```python
from build123d import *

# Parameters (mm, degrees)
F0_W     = 25.4
F0_H     = 127
F1_DEPTH = 12.7
F4_DEPTH = 12.7
F2_R     = 9.525
F5_DEPTH = 152.401


with BuildPart() as f1:
    # F0 (on Front) → F1 (new body, symmetric)
    with BuildSketch(Plane.XZ):
        with Locations((-3.775233, -0.143904)):
            Rectangle(F0_W, F0_H)
    extrude(amount=F1_DEPTH, both=True)

    # F3 (on Front) → F4 (join, symmetric)
    with BuildSketch(Plane.XZ):
        Polygon((-16.475233, 63.356096), (8.924767, 63.356096), (8.924767, 88.756096), align=None)
    extrude(amount=F4_DEPTH, both=True)

    # F2 (on face) → F5 (cut, through all)
    with BuildSketch(Plane(origin=(0, 0, -63.643904), x_dir=(1, 0, 0), z_dir=(0, 0, -1))):
        with Locations((-3.775233, 0)):
            Circle(F2_R)
    extrude(amount=-F5_DEPTH, mode=Mode.SUBTRACT)


solid = f1.part
```
Verification items for the finished model (mm, model axes). Give positions to 0.01 mm unless a question says otherwise; leave off trailing zeros. Loops run counter-clockwise (first coordinate to the right, second up) from the corner with the lowest first, then second, coordinate; pieces in that order, holes last.
1. Mould release check, pull along X, two halves, no side actions. Record for faces 1 (the cylindrical face through (5.31, -2.86, 9.92)), 2 (the flat face through (-3.6, 11.11, 76.23)), 3 (the flat face through (-4, 12.7, 14)): released by +X, released by -X, zero draft, split by the parting line, or undercut.
2. Thickness scan on line 1 (X direction, y = 0, z = 30.5); line 2 (Y direction, x = 1.25, z = -50); line 3 (Y direction, x = -4, z = -38.5). Record the ranges inside material, lowest first.
3. Section check B-B, the plane x = 0.75. Enter the section's corners in (y, z), then the cut area to 3 significant figures.
4. Section check A-A, the plane y = 3.75. Enter the section's corners in (x, z).
5. Go/stop test with a flat-tipped pin: pin 1 Ø8 at (x, y) = (-5.5, 2.5) entering from +Z. Record where the tip stops, or that it passes through.
Geometry says:
1. face 1: undercut
1. face 2: released by -X
1. face 3: zero draft
2. line 1: x = -16.48 to -13.3, 5.75 to 8.92
2. line 2: y = -12.7 to -8.09, 8.09 to 12.7
2. line 3: y = -12.7 to -9.52, 9.52 to 12.7
3. outline: (-12.7, -63.64) - (-8.38, -63.64) - (-8.38, 80.58) - (-12.7, 80.58) - close; (8.38, -63.64) - (12.7, -63.64) - (12.7, 80.58) - (8.38, 80.58) - close
3. area: 1,250 mm2
4. outline: (-16.48, -63.64) - (-12.53, -63.64) - (-12.53, 67.3) - (-16.48, 63.36) - close; (4.98, -63.64) - (8.92, -63.64) - (8.92, 88.76) - (4.98, 84.81) - close
5. pin 1: passes through
